```python
from build123d import *

# Parameters (mm, degrees)
SKETCH1_R           = 4.5
BOSS_EXTRUDE1_DEPTH = 7
SKETCH2_W           = 402.918493315
SKETCH2_H           = 212.645905023
CUT_EXTRUDE1_DEPTH  = 30
SKETCH3_R           = 3
CUT_EXTRUDE2_DEPTH  = 8.0000001


with BuildPart() as part:
    # Sketch1 → Boss-Extrude1 (new body)
    with BuildSketch(Plane.XY):
        with BuildLine():
            Line((22, -50), (-22, -50))
            Line((-22, -50), (-11, -305))
            ThreePointArc((-11, -305), (0, -315.535719965), (11, -305))
            Line((11, -305), (46.838884711, -72))
            Line((46.838884711, -72), (46.838884711, -60.421650598))
            add(Edge.make_bspline(
                [(46.838884711, -60.421650596), (43.068657692, -58.44092391), (40.423050609, -54.296947681), (40.046232129, -50)],
                knots=[0, 0, 0, 0, 0.425250978, 0.425250978, 0.425250978, 0.425250978], degree=3))
            Line((40.046232129, -50), (32, -50))
            ThreePointArc((32, -50), (30.828427125, -52.828427125), (28, -54))
            Line((28, -54), (26, -54))
            ThreePointArc((26, -54), (23.171572875, -52.828427125), (22, -50))
        make_face()
        with Locations((0, -305)):
            Circle(SKETCH1_R, mode=Mode.SUBTRACT)
    extrude(amount=BOSS_EXTRUDE1_DEPTH)

    # Sketch2 → Cut-Extrude1 (cut)
    with BuildSketch(Plane.XY.offset(7)):
        with Locations((44.983042226, -276.322952512)):
            Rectangle(SKETCH2_W, SKETCH2_H)
    extrude(amount=-CUT_EXTRUDE1_DEPTH, mode=Mode.SUBTRACT)

    # Sketch3 → Cut-Extrude2 (cut, through all)
    with BuildSketch(Plane.XY.offset(7)):
        with Locations((-7.159327661, -162)):
            Circle(SKETCH3_R)
        with Locations((7.840672339, -162)):
            Circle(SKETCH3_R)
        with Locations((22.840672339, -162)):
            Circle(SKETCH3_R)
    extrude(amount=-CUT_EXTRUDE2_DEPTH, mode=Mode.SUBTRACT)


solid = part.part
```
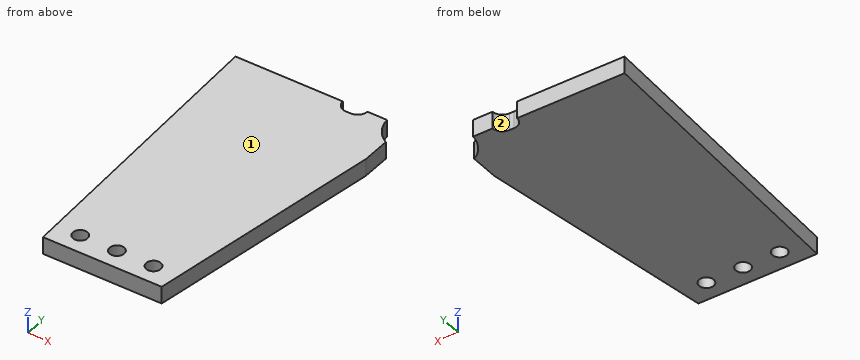
Verification items for the finished model (mm, model axes). Face numbers are marked on the shaded views. Coordinates: 2 decimals unless noted, no trailing zeros. Order: outer loops, then holes, each group sorted by start corner. A loop starts at its lowest first (then second) coordinate and runs counter-clockwise, first axis right, second up. Notation, with made-up numbers: (40.25, 45.5) -> (96.25, 45.5) arc R27 cw to (96.25, 82.5) -> close; hole circle Ø3 at (-30.75, -21). An arc over 180 degrees is marked (long way). Put each result on its own line as item: value. Start each with the question number.
1) Go/stop test with flat-tipped pins: pin 1 (0.6 mm diameter, centred on x = 27, z = 4.5, fed in from +Y); pin 2 (5 mm diameter, centred on x = 7.84, y = -162, fed in from -Z); pin 3 (2 mm diameter, centred on y = -127.5, z = 2, fed in from +X); pin 4 (1.5 mm diameter, centred on y = -138.5, z = 4, fed in from -X). Record where each tip stops, or that it passes through.
2) Cross-section at A-A (y = -162). Enter the section's corners in (x, z), plus the area to 3 significant figures.
3) Release check for a two-part mould opening along X. For the marked faces 1 and 2 record: pulls with the +X half, pulls with the -X half, needs draft (parallel to the pull), parting line crosses it, or undercut.
4) Cross-section at C-C (z = 5). State how many separate pieces and enclosed holes the cut face has, plus the area to 3 significant figures.
5) Material ranges on L1, parallel to X at y = -162, z = 1.5; L2, parallel to Y at x = 21.5, z = 3.25; L3, parallel to Y at x = -9, z = 3.5, recorded low to high.
6) Cross-section at D-D (x = 29.5). Enter the section's corners in (y, z), plus the area to 3 significant figures.
7) Cross-section at B-B (x = 7). Enter the section's corners in (y, z).
Geometry check:
1. pin 1: stops at y = -54
1. pin 2: passes through
1. pin 3: stops at x = 38.46
1. pin 4: stops at x = -18.21
2. outline: (-17.17, 0) -> (-10.16, 0) -> (-10.16, 7) -> (-17.17, 7) -> close; (-4.16, 0) -> (4.84, 0) -> (4.84, 7) -> (-4.16, 7) -> close; (10.84, 0) -> (19.84, 0) -> (19.84, 7) -> (10.84, 7) -> close; (25.84, 0) -> (33, 0) -> (33, 7) -> (25.84, 7) -> close
2. area: 225 mm^2
3. face 1: needs draft
3. face 2: undercut
4. separate pieces: 1
4. enclosed holes: 3
4. area: 7,050 mm^2
5. L1: x = -17.17 to -10.16, -4.16 to 4.84, 10.84 to 19.84, 25.84 to 33
5. L2: y = -170 to -164.68, -159.32 to -50
5. L3: y = -170 to -164.37, -159.63 to -50
6. outline: (-170, 0) -> (-53.71, 0) -> (-53.71, 7) -> (-170, 7) -> close
6. area: 814 mm^2
7. outline: (-170, 0) -> (-164.88, 0) -> (-164.88, 7) -> (-170, 7) -> close; (-159.12, 0) -> (-50, 0) -> (-50, 7) -> (-159.12, 7) -> close
